```python
from build123d import *

# Parameters (mm, degrees)
BOSS_EXTRUDE1_DEPTH      = 0.75
BOSS_EXTRUDE2_DEPTH      = 5
BOSS_EXTRUDE2_DEPTH_BACK = 1
SKETCH2_R                = 1.155


with BuildPart() as part:
    # Sketch1 → Boss-Extrude1 (new body)
    with BuildSketch(Plane.XY):
        with BuildLine():
            ThreePointArc((-2.116402116, 3.020870572), (-7.56, 0), (-2.116402116, -3.020870572))
            ThreePointArc((-2.116402116, -3.020870572), (0, -2.41510717), (2.116402116, -3.020870572))
            ThreePointArc((2.116402116, -3.020870572), (7.56, 0), (2.116402116, 3.020870572))
            ThreePointArc((2.116402116, 3.020870572), (0, 2.41510717), (-2.116402116, 3.020870572))
        make_face()
    boss_extrude1 = extrude(amount=BOSS_EXTRUDE1_DEPTH)

    # Sketch2 → Boss-Extrude2 (add, two sides: drawn at the far end of the back side and taken through both)
    with BuildSketch(Plane.XY.offset(0.75).offset(-BOSS_EXTRUDE2_DEPTH_BACK)):
        with Locations((-4, 0)):
            Circle(SKETCH2_R)
        with Locations((4, 0)):
            Circle(SKETCH2_R)
    extrude(amount=BOSS_EXTRUDE2_DEPTH + BOSS_EXTRUDE2_DEPTH_BACK)

    # Mirror1: Boss-Extrude1 across plane
    add(boss_extrude1.mirror(Plane.XY.offset(2.75)))


solid = part.part
```
Model file for the job. Use its own axes, mm. A direction names the side the tool comes from. Round coordinates to 2 decimals unless told otherwise and drop trailing zeros. Write each loop counter-clockwise with the first axis right and the second up, starting at its lowest first coordinate (ties: lowest second). Pieces come first, ordered by that corner, then holes. Notation, with made-up numbers: (43, -7) - (62, -7) arc R19 ccw to (62, 8) - close; hole circle Ø7 at (79.25, 47). An arc over 180 degrees is marked (long way). Use CSV: the item, a comma, the result in double quotes. Start each with the question number.
Item 1: Tool access for faces 1 (the face through (-7.56, 0.11, 5.13)), 2 (the face through (0, 0, 0.75)), 3 (the face through (0, 0, 5.5)): list every direction of +Z, -Z, +X, -X, +Y, -Y with a clear straight run to the whole face (end or side of a thin tool).
Item 2: Two-plate mould, pull along Z, no slides. Class faces 4 (the face through (0, 0, 4.75)), 5 (the face through (7.56, -0.11, 5.13)), 6 (the face through (0, 0, 0)): released by +Z, released by -Z, zero draft, split by the parting line, or undercut.
Item 3: Band-saw the part on D-D (y = -2.75). Write the cut outline in (x, z), and give its area (3 significant figures).
Item 4: Drill centre lines: L1, parallel to Z at x = 5, y = -2; L2, parallel to X at y = -2.75, z = 0.25; L3, parallel to Y at x = -5.25, z = 5.35. Where is each one in solid material? Low to high. Write a range as [from, to].
Item 5: Band-saw the part on A-A (x = -5.5). Write the cut outline in (y, z).
Item 6: Pin check, flat tips, straight feed: P1, Ø2, axis at x = 2, z = 4.5, coming from the -Y side; P2, Ø3, axis at y = 2, z = 1, coming from the +X side; P3, Ø1.5, axis at x = 4.5, z = 2, coming from the +Y side (3 decimals). Stop position of each tip, or through.
Item 7: Band-saw the part on C-C (z = 4.25). Write the cut outline in (x, y) (3 decimals), and give its area (3 significant figures).
Checked values:
1,face 1,"+Z, -Z"
1,face 2,"none"
1,face 3,"+Z"
2,face 4,"undercut"
2,face 5,"zero draft"
2,face 6,"released by -Z"
3,outline,"(-6.26, 0) - (-1.6, 0) - (-1.6, 0.75) - (-6.26, 0.75) - close; (-6.26, 4.75) - (-1.6, 4.75) - (-1.6, 5.5) - (-6.26, 5.5) - close; (1.6, 0) - (6.26, 0) - (6.26, 0.75) - (1.6, 0.75) - close; (1.6, 4.75) - (6.26, 4.75) - (6.26, 5.5) - (1.6, 5.5) - close"
3,area,"14.0 mm²"
4,L1,"z = [0, 0.75], [4.75, 5.5]"
4,L2,"x = [-6.26, -1.6], [1.6, 6.26]"
4,L3,"y = [-3.33, 3.33]"
5,outline,"(-3.23, 0) - (3.23, 0) - (3.23, 0.75) - (-3.23, 0.75) - close; (-3.23, 4.75) - (3.23, 4.75) - (3.23, 5.5) - (-3.23, 5.5) - close"
6,P1,"stops at y = -3.41"
6,P2,"stops at x = 7.52"
6,P3,"stops at y = 1.155"
7,outline,"circle Ø2.31 at (-4, 0); circle Ø2.31 at (4, 0)"
7,area,"8.38 mm²"
